from build123d import *

# Parameters (mm, degrees)
BOSS_EXTRUDE1_DEPTH = 3.175


with BuildPart() as part:
    # Sketch1 → Boss-Extrude1 (new body)
    with BuildSketch(Plane(origin=(0, 0, 0), x_dir=(1, 0, 0), z_dir=(0, 1, 0))):
        Polygon((-60.325, 68.834), (-85.725, 68.834), (-85.725, 43.434), (-88.9, 43.434), (-88.9, 18.034), (-85.725, 18.034), (-85.725, -18.034), (-88.9, -18.034), (-88.9, -43.434), (-85.725, -43.434), (-85.725, -68.834), (-60.325, -68.834), (-60.325, -65.659), (-34.925, -65.659), (-34.925, -68.834), (34.925, -68.834), (34.925, -65.659), (60.325, -65.659), (60.325, -68.834), (85.725, -68.834), (85.725, -43.434), (88.9, -43.434), (88.9, -18.034), (85.725, -18.034), (85.725, 18.034), (88.9, 18.034), (88.9, 43.434), (85.725, 43.434), (85.725, 68.834), (60.325, 68.834), (60.325, 65.659), (34.925, 65.659), (34.925, 68.834), (-34.925, 68.834), (-34.925, 65.659), (-60.325, 65.659), align=None)
        Polygon((-55.514400942, -56.134), (-9.641329679, -38.283634289), (9.641329679, -38.283634289), (55.514400942, -56.134), align=None, mode=Mode.SUBTRACT)
        Polygon((-27.151928737, -31.469819814), (-73.025, -49.320185525), (-73.025, -6.35), (-27.151928737, -6.35), align=None, mode=Mode.SUBTRACT)
        Polygon((0.606600295, 10.984138701), (-9.775001271, 16.993576732), (-9.775001271, 13.565679079), (-19.916767041, 13.565679079), (-19.916767041, 33.572617007), (-9.775001271, 33.572617007), (-9.775001271, 29.423230301), (9.770947304, 17.65448668), (9.770947304, 20.757112988), (19.912713073, 20.757112988), (19.912713073, 1.211164414), (9.770947304, 1.211164414), (9.770947304, 4.412046261), (2.366430033, 0), (9.770947304, -4.510587766), (9.770947304, -1.278178094), (19.912713073, -1.278178094), (19.912713073, -20.824126668), (9.770947304, -20.824126668), (9.770947304, -17.582605044), (-9.775001271, -29.404975555), (-9.775001271, -33.584778117), (-19.916767041, -33.584778117), (-19.916767041, -13.646113818), (-9.775001271, -13.646113818), (-9.775001271, -17.213122569), (0.606600295, -11.051152381), (-3.505546068, -8.798640388), (-3.505546068, -11.051152381), (-13.831707579, -11.051152381), (-13.831707579, 10.984138701), (-3.505546068, 10.984138701), (-3.505546068, 8.762018077), align=None, mode=Mode.SUBTRACT)
        Polygon((73.025, -6.35), (73.025, -49.320185525), (27.151928737, -31.469819814), (27.151928737, -6.35), align=None, mode=Mode.SUBTRACT)
        Polygon((-73.025, 49.320185525), (-27.151928737, 31.469819814), (-27.151928737, 6.35), (-73.025, 6.35), align=None, mode=Mode.SUBTRACT)
        Polygon((27.151928737, 6.35), (27.151928737, 31.469819814), (73.025, 49.320185525), (73.025, 6.35), align=None, mode=Mode.SUBTRACT)
        Polygon((9.641329679, 38.283634289), (-9.641329679, 38.283634289), (-55.514400942, 56.134), (55.514400942, 56.134), align=None, mode=Mode.SUBTRACT)
    extrude(amount=BOSS_EXTRUDE1_DEPTH)


solid = part.part
Read the model definition and answer for the solid it produces. Units are mm, in the model's axes. A direction names the side the tool comes from. Give positions to 0.01 mm unless a question says otherwise; leave off trailing zeros. Write each loop counter-clockwise with the first axis right and the second up, starting at its lowest first coordinate (ties: lowest second). Pieces come first, ordered by that corner, then holes. Notation, with made-up numbers: M 17,-9 L 62,-9 A33 ccw 62,26 Z; hole C -2.5,76 d9. An arc over 180 degrees is marked long. One line per item, written item: value. Start each with the question number.
(1) Flat-ended cylindrical pins translate along their axes: pin 1 Ø1.6 at (y, z) = (1.5, 68) entering from +X (3 decimals); pin 2 Ø1.6 at (x, y) = (-88, 2) entering from +Z; pin 3 Ø1 at (x, y) = (87, 1) entering from -Z. Find the tip coordinate at first contact, or state that the pin passes through.
(2) Find section B-B (z = 25). Determine the outline of the cut face in (x, y) (3 decimals).
(3) Find the intervals of material crossed by line 1 (X direction, y = 2.5, z = -29) (3 decimals); line 2 (Z direction, x = 7.5, y = 0.2); line 3 (Z direction, x = 38, y = 2.4), in increasing order.
(4) A tool of negligible diameter and unlimited length cuts with its end or side. For faces 3 (the flat face through (-21, 3.175, -1)), 4 (the flat face through (-50.41, 1.57, -40.52)), from which of +Z, -Z, +X, -X, +Y, -Y can it reach the whole face along a straight path? Write none if from no direction.
(5) Find section A-A (x = 70). Determine the outline of the cut face in (y, z) (3 decimals).
(6) Find section C-C (x = 6). Determine the outline of the cut face in (y, z) (3 decimals).
(7) Find section D-D (y = 1.7). Give the number of separate pieces and of enclosed holes in the cut face, plus the area to 3 significant figures.
(8) Determine the mould class of faces 1 (the flat face through (-4.7, 1.6, 14.2)), 2 (the flat face through (-21, 0, -1)) for opening direction X: pulls with the +X half, pulls with the -X half, needs draft (parallel to the pull), parting line crosses it, or undercut.
Results below:
1. pin 1: stops at x = 85.725
1. pin 2: stops at z = 43.43
1. pin 3: stops at z = -43.43
2. outline: M -88.9,0 L -73.025,0 L -73.025,3.175 L -88.9,3.175 Z; M -27.152,0 L -19.917,0 L -19.917,3.175 L -27.152,3.175 Z; M -2.492,0 L 27.152,0 L 27.152,3.175 L -2.492,3.175 Z; M 73.025,0 L 88.9,0 L 88.9,3.175 L 73.025,3.175 Z
3. line 1: x = -88.9 to -73.025, -27.152 to -19.917, -9.072 to 27.152, 73.025 to 88.9
3. line 2: z = -68.83 to -56.13, -38.28 to -19.02, -3.06 to 3.13, 18.96 to 38.28, 56.13 to 68.83
3. line 3: z = -65.66 to -56.13, -49.32 to -35.69, -6.35 to 6.35, 35.69 to 49.32, 56.13 to 65.66
4. face 3: +Z, -Z, +X, -X, +Y
4. face 4: +Y, -Y
5. outline: M 0,-68.834 L 3.175,-68.834 L 3.175,-48.143 L 0,-48.143 Z; M 0,-6.35 L 3.175,-6.35 L 3.175,6.35 L 0,6.35 Z; M 0,48.143 L 3.175,48.143 L 3.175,68.834 L 0,68.834 Z
6. outline: M 0,-68.834 L 3.175,-68.834 L 3.175,-56.134 L 0,-56.134 Z; M 0,-38.284 L 3.175,-38.284 L 3.175,-19.925 L 0,-19.925 Z; M 0,-2.165 L 3.175,-2.165 L 3.175,2.213 L 0,2.213 Z; M 0,19.863 L 3.175,19.863 L 3.175,38.284 L 0,38.284 Z; M 0,56.134 L 3.175,56.134 L 3.175,68.834 L 0,68.834 Z
7. separate pieces: 1
7. enclosed holes: 7
7. area: 13,300 mm^2
8. face 1: undercut
8. face 2: needs draft
